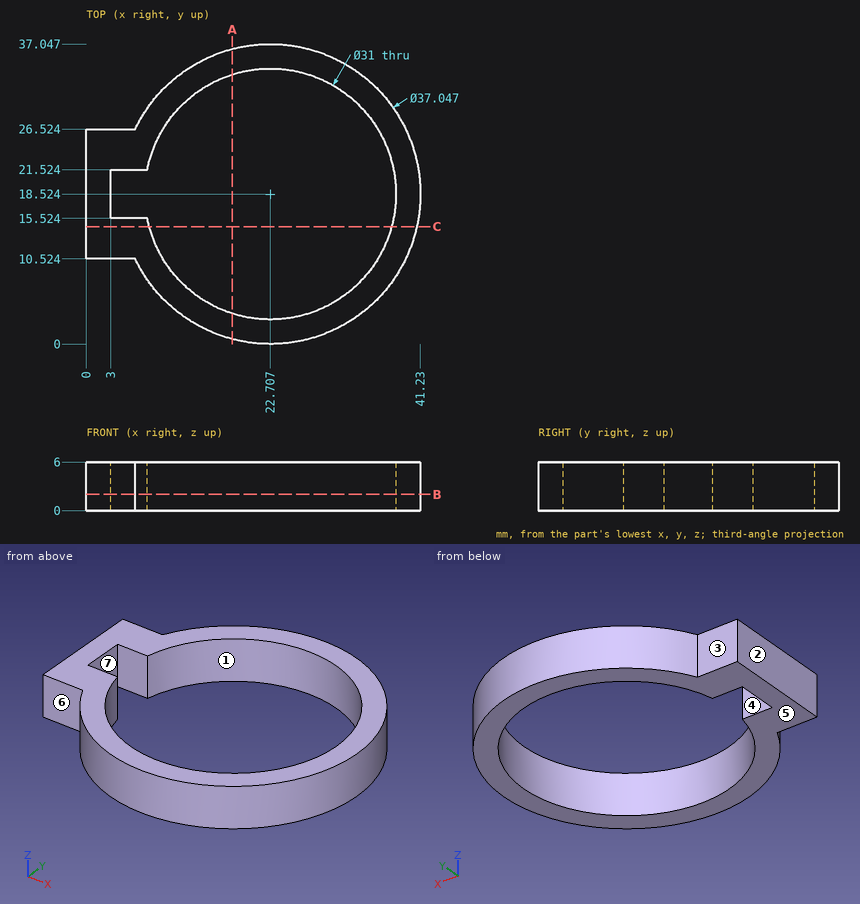
Could you check a few things on this drawing? It's one solid part, dimensions in mm from its lowest x, y, z. A direction names the side the tool comes from. Coordinates: 2 decimals unless noted, no trailing zeros. Write each loop counter-clockwise with the first axis right and the second up, starting at its lowest first coordinate (ties: lowest second). Pieces come first, ordered by that corner, then holes.
1) If we section it at C-C (y = 14.5): List the corners of the cut face in (x, z) for me (1 decimal), plus the area to 3 significant figures.
Filled in:
outline: (0, 0) - (7.7, 0) - (7.7, 6) - (0, 6) - close; (37.7, 0) - (40.8, 0) - (40.8, 6) - (37.7, 6) - close
area: 65.1 mm2
2) Which directions (+Z, -Z, +X, -X, +Y, -Y) give clear straight access to the entire face, cutting with the end or side of a thin tool? Please do the marked faces 5, 6 and 7.
Filled in:
face 5: -Z, +X, -X, +Y, -Y
face 6: +Z, -Z, -X, -Y
face 7: +Z, -Z
3) If we section it at B-B (z = 2): List the corners of the cut face in (x, y) for me, plus the area to 3 significant figures.
Filled in:
outline: (0, 10.52) - (6, 10.52) arc R18.52 ccw (long way) to (6, 26.52) - (0, 26.52) - close; hole (3, 15.52) - (7.5, 15.52) arc R15.5 ccw (long way) to (7.5, 21.52) - (3, 21.52) - close
area: 374 mm2
4) If we section it at A-A (x = 18): List the corners of the cut face in (y, z) for me (1 decimal).
Filled in:
outline: (0.6, 0) - (3.8, 0) - (3.8, 6) - (0.6, 6) - close; (33.3, 0) - (36.4, 0) - (36.4, 6) - (33.3, 6) - close
5) Thinking about a two-plate mould opening in X: for the marked faces 1, 2, 3 and 4, which applies, +X half, -X half, draft (parallel to the pull), parting line (faces both ways), or undercut?
Filled in:
face 1: undercut
face 2: -X half
face 3: draft
face 4: undercut
6) I'm going to push flat-ended pins straight in: pin 1 (1 mm diameter, centred on x = 7, z = 2.5, fed in from -Y) (1 decimal); pin 2 (3 mm diameter, centred on x = 3.5, z = 3, fed in from -Y); pin 3 (2.5 mm diameter, centred on x = 5, z = 3.5, fed in from +Y) (1 decimal). Where does each tip first touch, or does it pass through?
Filled in:
pin 1: stops at y = 7.9
pin 2: stops at y = 10.52
pin 3: stops at y = 27
7) If I drill on line 1 (X direction, y = 15, z = 1.95); line 2 (Y direction, x = 27.5, z = 3.75) (1 decimal); line 3 (Y direction, x = 5, z = 2.15), over which ranges is the centre line in solid material (lowest first)?
Filled in:
line 1: x = 0 to 7.61, 37.8 to 40.89
line 2: y = 0.6 to 3.8, 33.3 to 36.4
line 3: y = 10.52 to 15.52, 21.52 to 26.52
